Work out the finished part from the listing and answer in its coordinate system (mm). Face numbers are marked on the shaded views. Coordinates: 2 decimals unless noted, no trailing zeros. Loops run counter-clockwise (first coordinate to the right, second up) from the corner with the lowest first, then second, coordinate; pieces in that order, holes last.
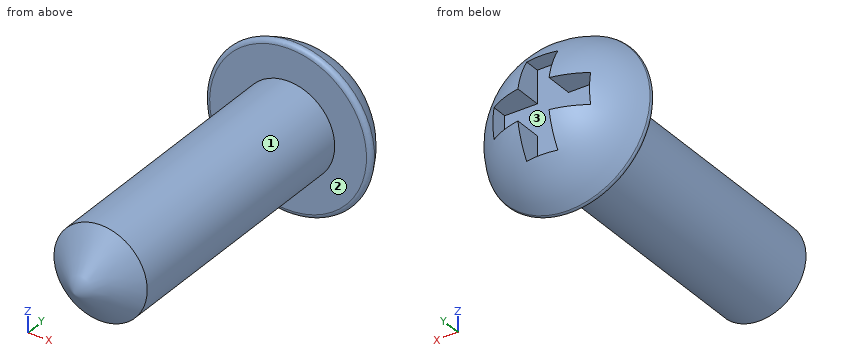
```python
from build123d import *

# Parameters (mm, degrees)
CONG_1_R                = 0.1
ENL_V_MAT_EXTRU_1_DEPTH = 0.5


with BuildPart() as part:
    # Esquisse1 → Révolution1 (revolve)
    with BuildSketch(Plane.XY, mode=Mode.PRIVATE) as r_volution1_sk:
        with BuildLine():
            Line((2, 0), (1.1, 0))
            Line((1.1, 0), (1.1, -6.4))
            Line((1.1, -6.4), (0, -7.302889311))
            Line((0, -7.302889311), (0, 1.382388101))
            ThreePointArc((0, 1.382388101), (1.215627087, 1.003157221), (2, 0))
        make_face()
    revolve(r_volution1_sk.sketch.rotate(Axis((0, 3.800054794, 0), (0, -1, 0)), 90), axis=Axis((0, 3.800054794, 0), (0, -1, 0)))

    # Congé1
    cong_1_edges = [part.edges().sort_by_distance(p)[0] for p in [
        (0, 0, -2),
    ]]
    fillet(cong_1_edges, radius=CONG_1_R)

    # Esquisse2 → Enlèv. mat.-Extru.1 (cut, symmetric)
    with BuildSketch(Plane(origin=(0, 1.15653742, 0), x_dir=(-1, 0, 0), z_dir=(0, 1, 0))):
        Polygon((-0.361948003, 1.140760916), (0.37159995, 1.140760916), (0.37159995, 0.37038863), (1.141972235, 0.37038863), (1.141972235, -0.363159322), (0.37159995, -0.363159322), (0.37159995, -1.133531608), (-0.361948003, -1.133531608), (-0.361948003, -0.363159322), (-1.132320288, -0.363159322), (-1.132320288, 0.37038863), (-0.361948003, 0.37038863), align=None)
    extrude(amount=ENL_V_MAT_EXTRU_1_DEPTH, both=True, mode=Mode.SUBTRACT)


solid = part.part
```
1. Determine the mould class of the marked faces 1, 2 and 3 for opening direction Z: released by +Z, released by -Z, zero draft, split by the parting line, or undercut.
2. A cutting plane is placed at A-A, the plane y = -4.5. Give the vertices of the cut face in (x, z).
3. Each of these flat-tipped pins is pushed along its axis until it touches: P1, Ø0.5, axis at y = 1, z = 1, coming from the -X side; P2, Ø0.5, axis at x = -0.5, y = 1, coming from the +Z side; P3, Ø0.7, axis at x = 0.5, y = 1, coming from the +Z side. Where does it stop, or does it pass through?
4. Straight lines are drawn through the part: probe 1 along Z at (x, y) = (0.7, -1.5); probe 2 along Y at (x, z) = (-0.55, 1.35); probe 3 along X at (y, z) = (0.75, -1.2). For each, find the intervals that lie inside material, in ascending order.
Answers below:
1. face 1: split by the parting line
1. face 2: zero draft
1. face 3: undercut
2. outline: circle Ø2.2 at (0, 0)
3. P1: stops at x = -1.2
3. P2: stops at z = 1.45
3. P3: stops at z = 1.55
4. probe 1: z = -0.85 to 0.85
4. probe 2: y = 0 to 0.81
4. probe 3: x = -0.93 to 0.93
